from build123d import *

# Parameters (mm, degrees)
SKETCH1_W           = 38.1
SKETCH1_H           = 31.75
BOSS_EXTRUDE1_DEPTH = 6.35
SKETCH2_W           = 12.7
SKETCH2_H           = 12.7
CUT_EXTRUDE1_DEPTH  = 50.99995


with BuildPart() as part:
    # Sketch1 → Boss-Extrude1 (new body)
    with BuildSketch(Plane(origin=(0, 0, 0), x_dir=(1, 0, 0), z_dir=(0, 1, 0))):
        with Locations((-19.05, 15.875)):
            Rectangle(SKETCH1_W, SKETCH1_H)
    extrude(amount=BOSS_EXTRUDE1_DEPTH)

    # Sketch2 → Cut-Extrude1 (cut, through all)
    with BuildSketch(Plane(origin=(0, 6.35, 0), x_dir=(1, 0, 0), z_dir=(0, 1, 0))):
        Polygon((-12.7, 26.67), (-27.305, 26.67), (-30.48, 23.495), (-30.48, 8.255), (-27.305, 5.08), (-12.7, 5.08), (-12.7, 9.525), (-12.7, 22.225), align=None)
        with Locations((-6.35, 15.875)):
            Rectangle(SKETCH2_W, SKETCH2_H)
        Polygon((0, 0), (0, 6.35), (-6.35, 0), align=None)
        Polygon((0, 31.75), (-6.35, 31.75), (0, 25.4), align=None)
        Polygon((-38.1, 6.35), (-31.75, 0), (-38.1, 0), align=None)
        Polygon((-38.1, 31.75), (-38.1, 25.4), (-32.371620034, 31.75), align=None)
    extrude(amount=-CUT_EXTRUDE1_DEPTH, mode=Mode.SUBTRACT)


solid = part.part
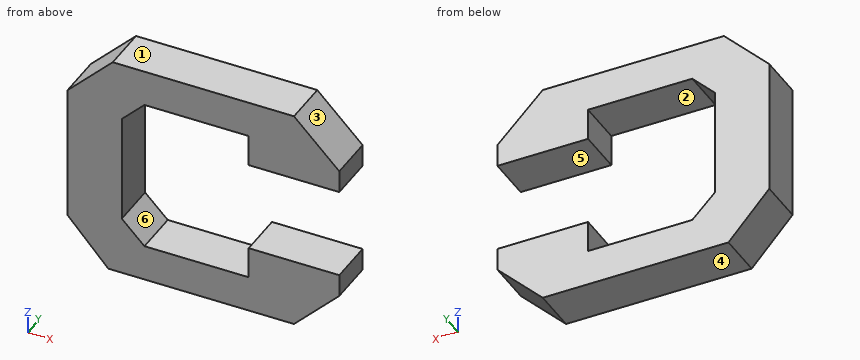
Geometry check sheet. Reference: the model listing, model coordinates, mm. Face numbers are marked on the shaded views. A direction names the side the tool comes from. Coordinates: 2 decimals unless noted, no trailing zeros. Write each loop counter-clockwise with the first axis right and the second up, starting at its lowest first coordinate (ties: lowest second). Pieces come first, ordered by that corner, then holes. Notation, with made-up numbers: (48, 24) -> (81, 24) arc R27 cw to (81, 61) -> close; hole circle Ø6 at (39, 62.25). An arc over 180 degrees is marked (long way). One line per question, with ' | ' between items.
1. Cross-section at A-A on z = -9. Record the cut outline in (x, y).
Answers:
outline: (-38.1, 0) -> (-30.48, 0) -> (-30.48, 6.35) -> (-38.1, 6.35) -> close; (-12.7, 0) -> (0, 0) -> (0, 6.35) -> (-12.7, 6.35) -> close
2. Depth check by flat-ended pin: pin 1 Ø1 at (x, y) = (-33, 0.5) entering from +Z; pin 2 Ø1.9 at (y, z) = (2, -16) entering from +X; pin 3 Ø1 at (x, z) = (-23, -28) entering from -Y. Enter the tip coordinate at first touch or a pass-through.
Answers:
pin 1: stops at z = -0.75 | pin 2: stops at x = -30.48 | pin 3: stops at y = 0
3. Thickness scan on probe 1 along Z at (x, y) = (-17, 3.25); probe 2 along Z at (x, y) = (-11, 3.5) (3 decimals); probe 3 along X at (y, z) = (4.5, -23). Record the ranges inside material, lowest first. Write a range as from..to.
Answers:
probe 1: z = -31.75..-26.67, -5.08..0 | probe 2: z = -31.75..-22.225, -9.525..0 | probe 3: x = -38.1..-30.48, -12.7..0
4. Draft check along X on the marked faces 1, 2 and 3. Enter one of: +X half, -X half, draft (parallel to the pull), parting line (faces both ways), or undercut.
Answers:
face 1: draft | face 2: undercut | face 3: +X half
5. Cross-section at D-D on z = -2. Record the cut outline in (x, y), and give its area (3 significant figures).
Answers:
outline: (-33.75, 0) -> (-4.35, 0) -> (-4.35, 6.35) -> (-33.75, 6.35) -> close | area: 187 mm²
6. Cross-section at B-B on x = -4. Record the cut outline in (y, z) (3 decimals).
Answers:
outline: (0, -29.4) -> (6.35, -29.4) -> (6.35, -22.225) -> (0, -22.225) -> close; (0, -9.525) -> (6.35, -9.525) -> (6.35, -2.35) -> (0, -2.35) -> close
7. Set-up check for the marked faces 4, 5 and 6: record each of +Z, -Z, +X, -X, +Y, -Y from which the full face is reachable in a straight line by a thin tool's end or side.
Answers:
face 4: -Z, +X, -X, +Y, -Y | face 5: +X, +Y, -Y | face 6: +Y, -Y
8. Cross-section at C-C on y = 3. Record the cut outline in (x, z) (3 decimals), and give its area (3 significant figures).
Answers:
outline: (-38.1, -25.4) -> (-32.372, -31.75) -> (-6.35, -31.75) -> (0, -25.4) -> (0, -22.225) -> (-12.7, -22.225) -> (-12.7, -26.67) -> (-27.305, -26.67) -> (-30.48, -23.495) -> (-30.48, -8.255) -> (-27.305, -5.08) -> (-12.7, -5.08) -> (-12.7, -9.525) -> (0, -9.525) -> (0, -6.35) -> (-6.35, 0) -> (-31.75, 0) -> (-38.1, -6.35) -> close | area: 596 mm²
